Build history of the part. All positions in model axes, mm. Face numbers are marked on the shaded views. A direction names the side the tool comes from. Give positions to 0.01 mm unless a question says otherwise; leave off trailing zeros. Order: outer loops, then holes, each group sorted by start corner. A loop starts at its lowest first (then second) coordinate and runs counter-clockwise, first axis right, second up. Notation, with made-up numbers: (57.5, 30) - (64.5, 30) arc R21 ccw to (64.5, 49) - close; hole circle Ø11 at (79, -6). An arc over 180 degrees is marked (long way). One line per item, written item: value.
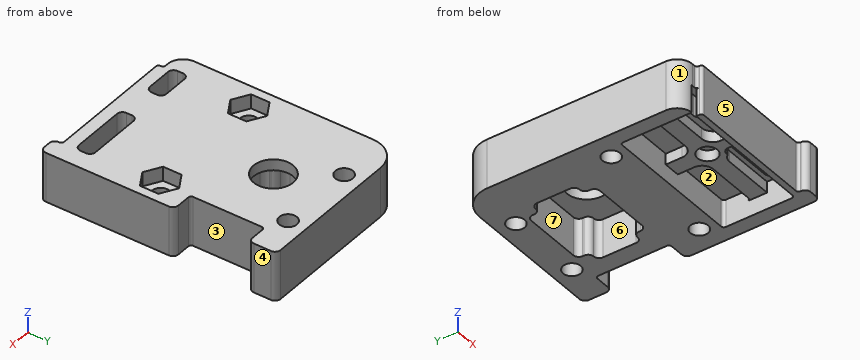
```python
from build123d import *

# Parameters (mm, degrees)
SKETCH_R        = 3.6
SKETCH_R_2      = 1.6
SKETCH_W        = 6.5
SKETCH_H        = 3
SKETCH_W_2      = 11.5
PAD_DEPTH       = 9
POCKET_DEPTH    = 2.6
POCKET001_DEPTH = 7
SKETCH003_W     = 25.7
SKETCH003_H     = 13
POCKET002_DEPTH = 3
SKETCH004_R     = 1.8
POCKET003_DEPTH = 2
FILLET_R        = 5
FILLET001_R     = 0.99
FILLET002_R     = 1
FILLET003_R     = 0.5


with BuildPart() as part:
    # Sketch → Pad (new body)
    with BuildSketch(Plane.XY):
        with BuildLine():
            Line((15.5, -31.15), (15.5, -6.75))
            Line((15.5, -6.75), (11.5, -6.75))
            Line((11.5, -6.75), (11.5, 6.75))
            Line((11.5, 6.75), (15.5, 6.75))
            Line((15.5, 6.75), (15.5, 11.85))
            Line((15.5, 11.85), (-15.5, 11.85))
            Line((-15.5, 11.85), (-15.5, -25.7))
            ThreePointArc((-15.5, -25.7), (-14.679899, -27.679899), (-12.7, -28.5))
            Line((-11.7, -28.5), (-12.7, -28.5))
            Line((-11.7, -29.55), (-11.7, -28.5))
            Line((-11.7, -29.55), (12.25, -29.55))
            Line((12.25, -29.55), (12.25, -31.15))
            Line((12.25, -31.15), (15.5, -31.15))
        make_face()
        Circle(SKETCH_R, mode=Mode.SUBTRACT)
        with Locations((-11, -12.5)):
            Circle(SKETCH_R_2, mode=Mode.SUBTRACT)
        with Locations((11, -12.5)):
            Circle(SKETCH_R_2, mode=Mode.SUBTRACT)
        with Locations((-6, 8.5)):
            Circle(SKETCH_R_2, mode=Mode.SUBTRACT)
        with Locations((8, 8.5)):
            Circle(SKETCH_R_2, mode=Mode.SUBTRACT)
        with Locations((-8.91, -25.81)):
            Rectangle(SKETCH_W, SKETCH_H, mode=Mode.SUBTRACT)
        with Locations((6.35, -25.81)):
            Rectangle(SKETCH_W_2, SKETCH_H, mode=Mode.SUBTRACT)
    extrude(amount=PAD_DEPTH)

    # Sketch001 (on Face28 of Pad) → Pocket (cut)
    with BuildSketch(Plane.XY.offset(9)):
        Polygon((-8.1, -14.174316), (-8.1, -10.825684), (-11, -9.151368), (-13.9, -10.825684), (-13.9, -14.174316), (-11, -15.848632), align=None)
        Polygon((13.9, -14.174316), (13.9, -10.825684), (11, -9.151368), (8.1, -10.825684), (8.1, -14.174316), (11, -15.848632), align=None)
    extrude(amount=-POCKET_DEPTH, mode=Mode.SUBTRACT)

    # Sketch002 → Pocket001 (cut)
    with BuildSketch(Plane(origin=(0, 0, 0), x_dir=(1, 0, 0), z_dir=(0, 0, -1))):
        Polygon((8.25, -4), (6.25, -4), (6.25, -6.25), (-6.25, -6.25), (-6.25, -4), (-8.25, -4), (-8.25, 4), (-6.25, 4), (-6.25, 6.25), (6.25, 6.25), (6.25, 4), (8.25, 4), align=None)
    extrude(amount=-POCKET001_DEPTH, mode=Mode.SUBTRACT)

    # Sketch003 → Pocket002 (cut)
    with BuildSketch(Plane(origin=(0, 0, 0), x_dir=(1, 0, 0), z_dir=(0, 0, -1))):
        with Locations((0, 22)):
            Rectangle(SKETCH003_W, SKETCH003_H)
    extrude(amount=-POCKET002_DEPTH, mode=Mode.SUBTRACT)

    # Sketch004 (on Face57 of Pocket002) → Pocket003 (cut)
    with BuildSketch(Plane(origin=(0, 0, 3), x_dir=(1, 0, 0), z_dir=(0, 0, -1))):
        with Locations((0, 22)):
            Circle(SKETCH004_R)
        with BuildLine():
            Line((1.5, 15.5), (12.85, 15.5))
            Line((12.85, 15.5), (12.85, 20.5))
            Line((12.85, 20.5), (3.5, 20.5))
            ThreePointArc((3.5, 20.5), (2.085786, 19.914214), (1.5, 18.5))
            Line((1.5, 18.5), (1.5, 15.5))
        make_face()
        with BuildLine():
            Line((-1.5, 15.5), (-12.85, 15.5))
            Line((-12.85, 15.5), (-12.85, 20.5))
            Line((-12.85, 20.5), (-3.5, 20.5))
            ThreePointArc((-1.5, 18.5), (-2.085786, 19.914214), (-3.5, 20.5))
            Line((-1.5, 18.5), (-1.5, 15.5))
        make_face()
        with BuildLine():
            Line((12.85, 23.5), (3.5, 23.5))
            ThreePointArc((1.5, 25.5), (2.085786, 24.085786), (3.5, 23.5))
            Line((1.5, 25.5), (1.5, 28.5))
            Line((1.5, 28.5), (12.85, 28.5))
            Line((12.85, 28.5), (12.85, 23.5))
        make_face()
        with BuildLine():
            Line((-12.85, 23.5), (-3.5, 23.5))
            ThreePointArc((-3.5, 23.5), (-2.085786, 24.085786), (-1.5, 25.5))
            Line((-1.5, 25.5), (-1.5, 28.5))
            Line((-1.5, 28.5), (-12.85, 28.5))
            Line((-12.85, 28.5), (-12.85, 23.5))
        make_face()
    extrude(amount=-POCKET003_DEPTH, mode=Mode.SUBTRACT)

    # Fillet
    fillet_edges = [part.edges().sort_by_distance(p)[0] for p in [
        (-15.5, 11.85, 4.5),
    ]]
    fillet(fillet_edges, radius=FILLET_R)

    # Fillet001
    fillet001_edges = [part.edges().sort_by_distance(p)[0] for p in [
        (6.25, 6.25, 3.5),
        (-6.25, 6.25, 3.5),
        (-6.25, 4, 3.5),
        (-8.25, 4, 3.5),
        (6.25, 4, 3.5),
        (8.25, 4, 3.5),
        (8.25, -4, 3.5),
        (6.25, -4, 3.5),
        (6.25, -6.25, 3.5),
        (-6.25, -6.25, 3.5),
        (-6.25, -4, 3.5),
        (-8.25, -4, 3.5),
    ]]
    fillet(fillet001_edges, radius=FILLET001_R)

    # Fillet002
    fillet002_edges = [part.edges().sort_by_distance(p)[0] for p in [
        (15.5, 11.85, 4.5),
        (15.5, 6.75, 4.5),
        (15.5, -6.75, 4.5),
        (15.5, -31.15, 4.5),
        (12.25, -31.15, 4.5),
        (12.1, -24.31, 7),
        (0.6, -24.31, 6),
        (12.1, -27.31, 7),
        (0.6, -27.31, 6),
        (-12.16, -24.31, 7),
        (-5.66, -24.31, 7),
        (-5.66, -27.31, 7),
        (-12.16, -27.31, 7),
    ]]
    fillet(fillet002_edges, radius=FILLET002_R)

    # Fillet003
    fillet003_edges = [part.edges().sort_by_distance(p)[0] for p in [
        (11.5, 6.75, 4.5),
        (11.5, -6.75, 4.5),
        (12.85, -15.5, 4),
        (12.85, -15.5, 1.5),
        (12.85, -20.5, 4),
        (-12.85, -15.5, 4),
        (-12.85, -15.5, 1.5),
        (-12.85, -23.5, 4),
        (-12.85, -20.5, 4),
        (-11.7, -29.55, 4.5),
        (12.85, -28.5, 1.5),
        (12.85, -28.5, 4),
        (12.25, -29.55, 4.5),
        (-11.7, -28.5, 7),
    ]]
    fillet(fillet003_edges, radius=FILLET003_R)


solid = part.part
```
(1) Pull direction Y, two halves, no side cores. Call the marked faces 4, 5, 6 and 7: +Y half, -Y half, draft (parallel to the pull), parting line (faces both ways), or undercut.
Completed:
face 4: draft
face 5: -Y half
face 6: undercut
face 7: undercut
(2) Slice it at D-D, the plane z = 1.5. Count the separate pieces of the cut face and the enclosed holes in it, and give its area (3 significant figures).
Completed:
separate pieces: 1
enclosed holes: 5
area: 669 mm²
(3) Slice it at A-A, the plane x = 0. Give the cut face in (y, z), and give its area (4 significant figures).
Completed:
outline: (-29.55, 0) - (-28.5, 0) - (-28.5, 3) - (-23.8, 3) - (-23.8, 5) - (-20.2, 5) - (-20.2, 3) - (-15.5, 3) - (-15.5, 0) - (-6.25, 0) - (-6.25, 7) - (-3.6, 7) - (-3.6, 9) - (-29.55, 9) - close; (3.6, 7) - (6.25, 7) - (6.25, 0) - (11.85, 0) - (11.85, 9) - (3.6, 9) - close
area: 224.5 mm²
(4) Slice it at C-C, the plane y = -22. Give the cut face in (x, z).
Completed:
outline: (-15.5, 0) - (-12.85, 0) - (-12.85, 3) - (-1.8, 3) - (-1.8, 5) - (1.8, 5) - (1.8, 3) - (12.85, 3) - (12.85, 0) - (15.5, 0) - (15.5, 9) - (-15.5, 9) - close
(5) Pin check, flat tips, straight feed: P1, Ø4, axis at x = 6, y = -20, coming from the -Z side; P2, Ø1.5, axis at y = 3, z = 6.5, coming from the +X side; P3, Ø1, axis at y = -6.5, z = 6, coming from the +X side; P4, Ø2.5, axis at x = -6, y = 8.5, coming from the -Z side. Stop position of each tip, or through.
Completed:
P1: z = 3
P2: x = 11.5
P3: x = 15.16
P4: through
(6) 3-axis set-ups, long thin cutter, end or side, ignore diameter. For the marked faces 1, 2 and 3: which of +Z, -Z, +X, -X, +Y, -Y reach the whole face in a straight line?
Completed:
face 1: +Z, -Z, -X, -Y
face 2: -Z
face 3: +Z, -Z, +X
(7) Drill centre lines: line 1 (X direction, y = -12.5, z = 1.75); line 2 (Y direction, x = 0, z = 3.95); line 3 (Y direction, x = 1.5, z = 1.5). Where is each one in solid material? Low to high.
Completed:
line 1: -15.5 to -12.6, -9.4 to 9.4, 12.6 to 15.5
line 2: -29.55 to -23.8, -20.2 to -6.25, 6.25 to 11.85
line 3: -29.55 to -28.5, -15.5 to -6.25, 6.25 to 11.85
(8) Slice it at B-B, the plane y = -12.5. Give the cut face in (x, z), and give its area (3 significant figures).
Completed:
outline: (-15.5, 0) - (-12.6, 0) - (-12.6, 6.4) - (-13.9, 6.4) - (-13.9, 9) - (-15.5, 9) - close; (-9.4, 0) - (9.4, 0) - (9.4, 6.4) - (8.1, 6.4) - (8.1, 9) - (-8.1, 9) - (-8.1, 6.4) - (-9.4, 6.4) - close; (12.6, 0) - (15.5, 0) - (15.5, 9) - (13.9, 9) - (13.9, 6.4) - (12.6, 6.4) - close
area: 208 mm²
